Solid Edge part; units mm, degrees
sketch "Sketch1" plane through (0, 0, 0) normal (0, -1, 0) x (1, 0, 0)
  line L0 (-16, -36) -> (16, -36)
  line L1 (16, -36) -> (16, 36)
  line L2 (16, 36) -> (-16, 36)
  line L3 (-16, 36) -> (-16, -36)
  line L4 (-20, -40) -> (20, -40)
  line L5 (20, -40) -> (20, 40)
  line L6 (20, 40) -> (-20, 40)
  line L7 (-20, 40) -> (-20, -40)
  dimension "D1" = 20
  dimension "D2" = 20
extrude "Protrusion1" add sketch "Sketch1" along normal mid plane 700
sketch "Sketch2" plane through (-20, 0, 0) normal (-1, 0, 0) x (0, -1, 0)
  line L0 (180.5, -40) -> (230.5, -40)
  line L1 (230.5, -40) -> (230.5, -35)
  line L2 (230.5, -35) -> (180.5, -35)
  line L3 (180.5, -35) -> (180.5, -40)
  line L4 (-299.5, -40) -> (-249.5, -40)
  line L5 (-249.5, -40) -> (-249.5, -35)
  line L6 (-249.5, -35) -> (-299.5, -35)
  line L7 (-299.5, -35) -> (-299.5, -40)
  dimension "D1" = 249.5
  dimension "D2" = 249.5
  dimension "D3" = 230.5
  dimension "D4" = 180.5
extrude "Cutout1" cut sketch "Sketch2" against normal through all
chamfer "Chamfer1" distance 2 angle 45 2 edges at (0, -230.5, -40) (0, -180.5, -40)
chamfer "Fase_5" distance 2 angle 45 2 edges at (0, 249.5, -40) (0, 299.5, -40)
chamfer "Fase_6" distance 2 angle 45 2 edges at (20, 274.5, -35) (-20, 274.5, -35)
chamfer "Fase_7" distance 2 angle 45 2 edges at (20, -205.5, -35) (-20, -205.5, -35)
sketch "Sketch3" plane through (20, 0, 0) normal (1, 0, 0) x (0, 1, 0)
  circle A0 centre (-216, -19) radius 4
  circle A1 centre (-120, -19) radius 4
  circle A2 centre (-102, -19) radius 4
  circle A3 centre (-234, -19) radius 4
  dimension "D1" = 120
  dimension "D2" = 234
  dimension "D3" = 216
  dimension "D4" = 234
extrude "Cutout2" cut sketch "Sketch3" against normal through all
sketch "Sketch4" plane through (-20, 0, 0) normal (-1, 0, 0) x (0, -1, 0)
  circle A0 centre (-126, 10) radius 3.5
  circle A1 centre (34, 10) radius 3.5
  dimension "D1" = 126
  dimension "D2" = 126
extrude "Cutout3" cut sketch "Sketch4" against normal through all
sketch "Sketch5" plane through (-20, 0, 0) normal (-1, 0, 0) x (0, -1, 0)
  line L0 (350, 40) -> (313.5, 40)
  line L1 (313.5, 40) -> (313.5, 36)
  line L2 (313.5, 36) -> (346, 36)
  line L3 (346, 36) -> (346, 32)
  line L4 (346, 32) -> (350, 32)
  line L5 (350, 32) -> (350, 40)
  dimension "D1" = 350
  dimension "D2" = 313.5
  dimension "D3" = 346
  dimension "D4" = 346
extrude "Cutout4" cut sketch "Sketch5" against normal through all
mirror "Mirror1" about plane through (0, 0, 0) normal (0, 0, 1) of "Cutout4"
mirror "Mirror2" about plane through (0, 0, 0) normal (0, -1, 0) of "Cutout4", "Mirror1"
sketch "Sketch6" plane through (-20, 0, 0) normal (-1, 0, 0) x (0, 1, 0)
  circle A0 centre (-330, 0) radius 3
  circle A1 centre (-300, -25) radius 3
  circle A2 centre (-300, 25) radius 3
  dimension "D1" = 330
extrude "Cutout5" cut sketch "Sketch6" against normal through all
mirror "Mirror3" about plane through (0, 0, 0) normal (0, -1, 0) of "Cutout5"
properties material "Aluminium, 6061-T6"
Input: part model. Units: mm. Frame: model coordinates. A direction names the side the tool comes from. Round coordinates to 2 decimals unless told otherwise and drop trailing zeros. Order: outer loops, then holes, each group sorted by start corner. A loop starts at its lowest first (then second) coordinate and runs counter-clockwise, first axis right, second up. Notation, with made-up numbers: (42.25, -6.75) - (96.25, -6.75) arc R14 cw to (96.25, 9.25) - close; hole circle Ø3 at (62, 44.25). An arc over 180 degrees is marked (long way). Use a Markdown table: item, result.
1. Access query for faces 4 (the face through (-16, 5, 1)), 5 (the face through (-20, 5, 1)). Directions: +Z, -Z, +X, -X, +Y, -Y. A direction counts if a zero-diameter tool reaches every point of the face in a straight line with its end or side. Return the directions, or none.
Evaluation:
| item | result |
|---|---|
| face 4 | +Y, -Y |
| face 5 | +Z, -Z, -X, +Y, -Y |
2. Section A-A on x = -1.5. Return the cut outline in (y, z), then the cut area to 3 significant figures.
Evaluation:
| item | result |
|---|---|
| outline | (-313.5, -40) - (-232.5, -40) - (-230.5, -38) - (-230.5, -36) - (-313.5, -36) - close; (-313.5, 36) - (313.5, 36) - (313.5, 40) - (-313.5, 40) - close; (-180.5, -38) - (-178.5, -40) - (247.5, -40) - (249.5, -38) - (249.5, -36) - (-180.5, -36) - close; (299.5, -38) - (301.5, -40) - (313.5, -40) - (313.5, -36) - (299.5, -36) - close |
| area | 4,610 mm^2 |
3. Section B-B on y = 266.5. Return the cut outline in (x, z).
Evaluation:
| item | result |
|---|---|
| outline | (-20, -33) - (-18, -35) - (-16, -35) - (-16, 36) - (16, 36) - (16, -35) - (18, -35) - (20, -33) - (20, 40) - (-20, 40) - close |
4. Mould query, pull axis X, two halves, no side actions, for faces 1 (the face through (0, 38, -36)), 2 (the face through (0, 37, -40)), 3 (the face through (20, 5, -1)). Classes: +X half, -X half, draft (parallel to the pull), parting line (faces both ways), or undercut.
Evaluation:
| item | result |
|---|---|
| face 1 | undercut |
| face 2 | draft |
| face 3 | +X half |
5. Material intervals for probe 1 along Z at (x, y) = (-17, -102); probe 2 along X at (y, z) = (79, 15); probe 3 along Y at (x, z) = (-17, 25), sorted ascending.
Evaluation:
| item | result |
|---|---|
| probe 1 | -40 to -23, -15 to 40 |
| probe 2 | -20 to -16, 16 to 20 |
| probe 3 | -350 to -303, -297 to 297, 303 to 350 |
6. First-contact query: pin 1 (3.5 mm diameter, centred on y = 330, z = 0, fed in from -X); pin 2 (2 mm diameter, centred on x = 18.5, y = -348, fed in from +Z); pin 3 (3 mm diameter, centred on x = 17, y = 335, fed in from -Z); pin 4 (2 mm diameter, centred on x = 3, z = 38.5, fed in from -Y). Flat tips, straight axial feed; report the tip coordinate or a pass-through.
Evaluation:
| item | result |
|---|---|
| pin 1 | through |
| pin 2 | z = 32 |
| pin 3 | z = -36 |
| pin 4 | y = -313.5 |
